```python
from build123d import *

# Parameters (mm, degrees)
F0_W     = 105.568755
F0_H     = 92.456006
F1_DEPTH = 12.7
F2_W     = 105.568755
F2_H     = 92.456006
F3_DEPTH = 12.7
F5_DEPTH = 25.4
F7_DEPTH = 25.4


with BuildPart() as f1:
    # F0 (on Right) → F1 (new body)
    with BuildSketch(Plane.YZ):
        with Locations((0.889001, 0.333376)):
            Rectangle(F0_W, F0_H)
    extrude(amount=F1_DEPTH)

    # F2 (on face) → F3 (join)
    with BuildSketch(Plane(origin=(0, 0, 0), x_dir=(0, -1, 0), z_dir=(-1, 0, 0))):
        with Locations((-0.889001, 0.333376)):
            Rectangle(F2_W, F2_H)
    extrude(amount=F3_DEPTH)

    # F4 (on face) → F5 (join)
    with BuildSketch(Plane(origin=(-12.7, 0, 0), x_dir=(0, -1, 0), z_dir=(-1, 0, 0))):
        Polygon((51.895376, -45.894627), (0, 0), (0, 46.561379), (-53.673379, 46.561379), (-53.673379, -45.894627), align=None)
    extrude(amount=F5_DEPTH)

    # F6 (on face) → F7 (join)
    with BuildSketch(Plane.YZ.offset(12.7)):
        Polygon((0, 46.561379), (0, 0), (-51.895376, -45.894627), (53.673379, -45.894627), (53.673379, 46.561379), align=None)
    extrude(amount=F7_DEPTH)


solid = f1.part
```
Work out the finished part from the listing and answer in its coordinate system (mm). A direction names the side the tool comes from. Round coordinates to 2 decimals unless told otherwise and drop trailing zeros. Write each loop counter-clockwise with the first axis right and the second up, starting at its lowest first coordinate (ties: lowest second). Pieces come first, ordered by that corner, then holes. Notation, with made-up numbers: (33, 28) -> (48, 28) arc R23 ccw to (48, 52) -> close; hole circle Ø3 at (-40, -23). An arc over 180 degrees is marked (long way). Write each question's results on one line, items separated by ' | '.
Q1. Section B-B, the plane y = -6 is taken. Write down the section's boundary in (x, z), then the cut area to 3 significant figures.
Data:
outline: (-38.1, -45.89) -> (38.1, -45.89) -> (38.1, -5.31) -> (12.7, -5.31) -> (12.7, 46.56) -> (-12.7, 46.56) -> (-12.7, -5.31) -> (-38.1, -5.31) -> close | area: 4,410 mm^2
Q2. Section C-C, the plane x = 23 is taken. Write down the section's boundary in (y, z).
Data:
outline: (-51.9, -45.89) -> (53.67, -45.89) -> (53.67, 46.56) -> (0, 46.56) -> (0, 0) -> close
Q3. Straight lines are drawn through the part: line 1 along X through (y, z) = (-23.5, -19.5); line 2 along Y through (x, z) = (32, 23.5); line 3 along Y through (x, z) = (17.5, -38). For each, find the intervals that lie inside material, in ascending order. Write a range as [from, to].
Data:
line 1: [-12.7, 12.7] | line 2: [0, 53.67] | line 3: [-42.97, 53.67]
Q4. Which of the six approach directions +Z, -Z, +X, -X, +Y, -Y give full straight-line access (tool end or side, diameter ignored) to faces 1 (the flat face through (0, 53.673, 0)), 2 (the flat face through (-25.22, -26.31, -23.27)), 3 (the flat face through (25, 0, 24))?
Data:
face 1: +Z, -Z, +X, -X, +Y | face 2: +Z, -X, -Y | face 3: +Z, +X, -Y
Q5. Flat-ended cylindrical pins translate along their axes: P1, Ø2, axis at x = -14, y = -15, coming from the +Z side; P2, Ø12, axis at y = -25, z = -10.5, coming from the -X side; P3, Ø20.5, axis at x = 26, z = 18, coming from the -Y side. Find the tip coordinate at first contact, or state that the pin passes through.
Data:
P1: z = -12.38 | P2: x = -12.7 | P3: y = 0
Q6. Section D-D, the plane z = -21 is taken. Write down the section's boundary in (x, y).
Data:
outline: (-38.1, -23.75) -> (-12.7, -23.75) -> (-12.7, -51.9) -> (12.7, -51.9) -> (12.7, -23.75) -> (38.1, -23.75) -> (38.1, 53.67) -> (-38.1, 53.67) -> close
Q7. Section A-A, the plane z = 9 is taken. Write down the section's boundary in (x, y), then the cut area to 3 significant figures.
Data:
outline: (-38.1, 0) -> (-12.7, 0) -> (-12.7, -51.9) -> (12.7, -51.9) -> (12.7, 0) -> (38.1, 0) -> (38.1, 53.67) -> (-38.1, 53.67) -> close | area: 5,410 mm^2
